Check sheet for the modelled part. Datum: model origin and axes. Units: mm. A direction names the side the tool comes from. Round coordinates to 2 decimals unless told otherwise and drop trailing zeros. Loops run counter-clockwise (first coordinate to the right, second up) from the corner with the lowest first, then second, coordinate; pieces in that order, holes last. Notation, with made-up numbers: (61.5, 56.25) -> (69.5, 56.25) arc R24 cw to (69.5, 69.25) -> close; hole circle Ø9 at (74, -38). An arc over 180 degrees is marked (long way). Return JSON: item names as keys, results as strings.
from build123d import *

# Parameters (mm, degrees)
BOX009_W                  = 41
BOX009_H                  = 42
BOX009_DEPTH              = 40
BOX008_W                  = 7
BOX008_H                  = 17
BOX008_DEPTH              = 10
CYLINDER004_R             = 2.5
CYLINDER004_DEPTH         = 25
CYLINDER005_R             = 2.5
CYLINDER005_DEPTH         = 4
BOX012_W                  = 45
BOX012_H                  = 3
BOX012_DEPTH              = 8
BOX011_W                  = 3
BOX011_H                  = 50
BOX011_DEPTH              = 8
BOX010_W                  = 45
BOX010_H                  = 50
BOX010_DEPTH              = 3
FUSION005_ROLL_ANGLE      = -90
FUSION005_PLACEMENT_ANGLE = 90


with BuildPart() as base_motor001:
    # Box009 → Box009 (new body)
    with BuildSketch(Plane(origin=(4, 4, 0), x_dir=(1, 0, 0), z_dir=(0, 0, 1))):
        with Locations((20.5, 21)):
            Rectangle(BOX009_W, BOX009_H)
    extrude(amount=BOX009_DEPTH)


with BuildPart() as obj1:
    # Box008 → Box008 (new body)
    with BuildSketch(Plane(origin=(45, 16.5, 0), x_dir=(1, 0, 0), z_dir=(0, 0, 1))):
        with Locations((3.5, 8.5)):
            Rectangle(BOX008_W, BOX008_H)
    extrude(amount=BOX008_DEPTH)


with BuildPart() as motor001:
    # Cylinder004 → Cylinder004 (new body)
    with BuildSketch(Plane(origin=(25, 25, 38), x_dir=(1, 0, 0), z_dir=(0, 0, 1))):
        Circle(CYLINDER004_R)
    extrude(amount=CYLINDER004_DEPTH)

    # Fusion007: union base motor001, obj1
    add(base_motor001.part)
    add(obj1.part)


with BuildPart() as obj2:
    # Cylinder005 → Cylinder005 (new body)
    with BuildSketch(Plane(origin=(10, 10, 43), x_dir=(1, 0, 0), z_dir=(0, 0, 1))):
        Circle(CYLINDER005_R)
    extrude(amount=CYLINDER005_DEPTH)


with BuildPart() as obj3:
    # Link009 base: copy of obj2
    add(obj2.part)


with BuildPart() as obj3_1:
    # Link009 placement: moved
    add(obj3.part.moved(Location((30, 30, 0))))


with BuildPart() as obj4:
    # Link010 base: copy of obj2
    add(obj2.part)


with BuildPart() as obj4_1:
    # Link010 placement: moved
    add(obj4.part.moved(Location((30, 0, 0))))


with BuildPart() as obj5:
    # Link007 base: copy of obj2
    add(obj2.part)


with BuildPart() as obj5_1:
    # Link007 placement: moved
    add(obj5.part.moved(Location((0, 30, 0))))


with BuildPart() as obj6:
    # Box012 → Box012 (new body)
    with BuildSketch(Plane.XY.offset(32)):
        with Locations((22.5, 1.5)):
            Rectangle(BOX012_W, BOX012_H)
    extrude(amount=BOX012_DEPTH)


with BuildPart() as lateral_der001:
    # Link008 base: copy of obj6
    add(obj6.part)


with BuildPart() as lateral_der001_1:
    # Link008 placement: moved
    add(lateral_der001.part.moved(Location((0, 47, 0))))


with BuildPart() as obj7:
    # Box011 → Box011 (new body)
    with BuildSketch(Plane.XY.offset(32)):
        with Locations((1.5, 25)):
            Rectangle(BOX011_W, BOX011_H)
    extrude(amount=BOX011_DEPTH)


with BuildPart() as obj8:
    # Box010 → Box010 (new body)
    with BuildSketch(Plane.XY.offset(40)):
        with Locations((22.5, 25)):
            Rectangle(BOX010_W, BOX010_H)
    extrude(amount=BOX010_DEPTH)

    # Fusion006: union obj6, lateral der001, obj7
    add(obj6.part)
    add(lateral_der001_1.part)
    add(obj7.part)

    # Fusion005: union motor001, obj3, obj4, obj5, obj2
    add(motor001.part)
    add(obj3_1.part)
    add(obj4_1.part)
    add(obj5_1.part)
    add(obj2.part)


with BuildPart() as obj8_1:
    # Fusion005 roll: moved
    add(obj8.part.rotate(Axis((0, 0, 0), (1, 0, 0)), FUSION005_ROLL_ANGLE))


with BuildPart() as obj8_2:
    # Fusion005 placement: moved
    add(obj8_1.part.moved(Location((152, -22.5, 55))).rotate(Axis((152, -22.5, 55), (0, 0, 1)), FUSION005_PLACEMENT_ANGLE))


solid = obj8_2.part
Q1. Go/stop test with flat-tipped pins: pin 1 (1 mm diameter, centred on y = 7.5, z = 11.5, fed in from -X); pin 2 (2.5 mm diameter, centred on x = 114, z = 36, fed in from +Y); pin 3 (3 mm diameter, centred on y = -14.5, z = 12, fed in from -X). Record where each tip stops, or that it passes through.
Results list:
{"pin 1": "x = 109", "pin 2": "y = 22.5", "pin 3": "x = 105"}
Q2. Material ranges on line 1 (Z direction, x = 117, y = 3); line 2 (Y direction, x = 116.5, z = 20.5); line 3 (X direction, y = -1, z = 10), recorded low to high.
Results list:
{"line 1": "5 to 8, 9 to 51, 52 to 55", "line 2": "-22.5 to -19.5, -18.5 to 22.5", "line 3": "109 to 152"}
Q3. Section check C-C (y = 17.5). Record the boundary of the cut face in (x, z).
Results list:
{"outline": "(105, 12.5) -> (109, 12.5) -> (109, 5) -> (120, 5) -> (120, 8) -> (112, 8) -> (112, 9) -> (152, 9) -> (152, 51) -> (112, 51) -> (112, 52) -> (120, 52) -> (120, 55) -> (109, 55) -> (109, 47.5) -> (105, 47.5) -> (105, 42.5) -> (109, 42.5) -> (109, 17.5) -> (105, 17.5) -> close"}
Q4. Tool access check on faces 5 (the flat face through (116, -19.5, 30)), 6 (the flat face through (116, 1, 8)), 7 (the flat face through (142, 26, 30)), 8 (the flat face through (147, 26, 21.5)). Record the directions out of +Z, -Z, +X, -X, +Y, -Y that give a thin tool (end or side, any length) a straight path to the whole face; none if there is none.
Results list:
{"face 5": "+X", "face 6": "+X, +Y", "face 7": "+Z, -Z, -X, +Y", "face 8": "-Z, +X, -X, +Y"}
Q5. Draft check along Z on faces 1 (the cylindrical face through (107, 16, 47)), 2 (the flat face through (115, -22.5, 30)), 3 (the flat face through (115, 0, 5)), 4 (the flat face through (147, 26, 38.5)). Enter one of: released by +Z, released by -Z, zero draft, split by the parting line, or undercut.
Results list:
{"face 1": "undercut", "face 2": "zero draft", "face 3": "released by -Z", "face 4": "released by +Z"}
Q6. Section check B-B (z = 43.5). Record the boundary of the cut face in (x, y), then the cut area to 3 significant figures.
Results list:
{"outline": "(105, -14.5) -> (109, -14.5) -> (109, -22.5) -> (120, -22.5) -> (120, -19.5) -> (112, -19.5) -> (112, -18.5) -> (152, -18.5) -> (152, 22.5) -> (109, 22.5) -> (109, 19.5) -> (105, 19.5) -> (105, 15.5) -> (109, 15.5) -> (109, -10.5) -> (105, -10.5) -> close", "area": "1,830 mm^2"}
Q7. Section check A-A (x = 113). Record the boundary of the cut face in (y, z).
Results list:
{"outline": "(-22.5, 5) -> (22.5, 5) -> (22.5, 8) -> (-19.5, 8) -> (-19.5, 52) -> (22.5, 52) -> (22.5, 55) -> (-22.5, 55) -> close; (-18.5, 9) -> (22.5, 9) -> (22.5, 51) -> (-18.5, 51) -> close"}
Q8. Section check D-D (z = 30). Record the boundary of the cut face in (x, y), then the cut area to 3 significant figures.
Results list:
{"outline": "(89, 0) -> (109, 0) -> (109, -22.5) -> (120, -22.5) -> (120, -19.5) -> (112, -19.5) -> (112, -18.5) -> (152, -18.5) -> (152, 29.5) -> (142, 29.5) -> (142, 22.5) -> (109, 22.5) -> (109, 5) -> (89, 5) -> close", "area": "1,970 mm^2"}
